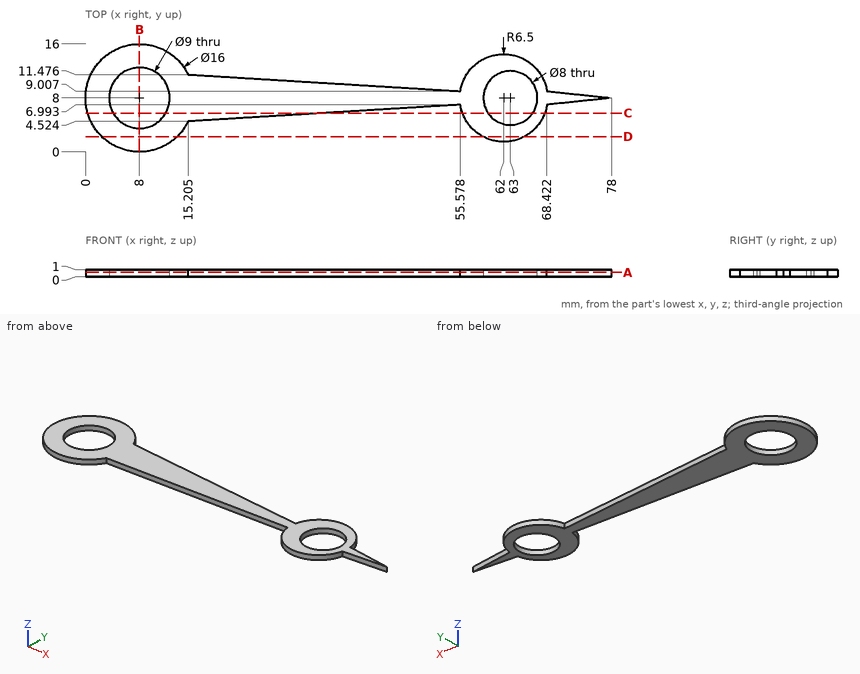
Verification items for this drawing (mm, ordinates from the low corner). Coordinates: 2 decimals unless noted, no trailing zeros. Write each loop counter-clockwise with the first axis right and the second up, starting at its lowest first coordinate (ties: lowest second). Pieces come first, ordered by that corner, then holes. Notation, with made-up numbers: M 23.25,30 L 33.25,30 A10 ccw 33.25,39 Z; hole C 47.5,27.25 d5. An arc over 180 degrees is marked long. Use CSV: the item, a comma, the result in double quotes.
Q1. Section check B-B, the plane x = 8. Enter the section's corners in (y, z).
Computed values:
outline,"M 0,0 L 3.5,0 L 3.5,1 L 0,1 Z; M 12.5,0 L 16,0 L 16,1 L 12.5,1 Z"
Q2. Thickness scan on line 1 along Y through (x, z) = (8, 0.75); line 2 along X through (y, z) = (2, 0.7) (1 decimal); line 3 along Y through (x, z) = (64.5, 0.95). Record the ranges inside material, lowest first. Write a range as [from, to].
Computed values:
line 1,"[0, 3.5], [12.5, 16]"
line 2,"[2.7, 13.3], [59.5, 64.5]"
line 3,"[2, 4.29], [11.71, 14]"
Q3. Section check C-C, the plane y = 5.75. Enter the section's corners in (x, z).
Computed values:
outline,"M 0.32,0 L 4.1,0 L 4.1,1 L 0.32,1 Z; M 11.9,0 L 35.25,0 L 35.25,1 L 11.9,1 Z; M 55.9,0 L 59.69,0 L 59.69,1 L 55.9,1 Z; M 66.31,0 L 68.1,0 L 68.1,1 L 66.31,1 Z"
Q4. Section check A-A, the plane z = 0.65. Enter the section's corners in (x, y) (1 decimal).
Computed values:
outline,"M 15.2,4.5 L 55.6,7 A6.5 ccw 68.4,7 L 78,8 L 68.4,9 A6.5 ccw 55.6,9 L 15.2,11.5 A8 ccw long Z; hole C 8,8 d9; hole C 63,8 d8"
Q5. Section check D-D, the plane y = 2.25. Enter the section's corners in (x, z), and give its area (3 significant figures).
Computed values:
outline,"M 2.44,0 L 13.56,0 L 13.56,1 L 2.44,1 Z; M 58.97,0 L 65.03,0 L 65.03,1 L 58.97,1 Z"
area,"17.2 mm²"
Q6. Go/stop test with a flat-tipped pin: P1, Ø9, axis at x = 63, y = 8, coming from the +Z side. Record where the tip stops, or that it passes through.
Computed values:
P1,"z = 1"
